Build history of the part. All positions in model axes, mm. A direction names the side the tool comes from. Coordinates: 2 decimals unless noted, no trailing zeros. Order: outer loops, then holes, each group sorted by start corner. A loop starts at its lowest first (then second) coordinate and runs counter-clockwise, first axis right, second up. Notation, with made-up numbers: (52.5, -30) - (102.5, -30) arc R33 ccw to (102.5, -1) - close; hole circle Ø1 at (82.25, -35.75). An arc over 180 degrees is marked (long way). Return JSON: item names as keys, results as strings.
from build123d import *

# Parameters (mm, degrees)
BOSS_EXTRUDE1_DEPTH      = 203.2
BOSS_EXTRUDE1_DEPTH_BACK = 203.2
SKETCH1_W                = 25.4
SKETCH1_H                = 25.4
SKETCH1_W_2              = 22.225
SKETCH1_H_2              = 22.225
FILLET1_R                = 0.79375
CUT_EXTRUDE1_DEPTH       = 206.174779152


with BuildPart() as part:
    # Sketch1 → Boss-Extrude1 (new, two sides: drawn at the far end of the back side and taken through both)
    with BuildSketch(Plane.XY.offset(-BOSS_EXTRUDE1_DEPTH_BACK)):
        Rectangle(SKETCH1_W, SKETCH1_H)
        Rectangle(SKETCH1_W_2, SKETCH1_H_2, mode=Mode.SUBTRACT)
    extrude(amount=BOSS_EXTRUDE1_DEPTH + BOSS_EXTRUDE1_DEPTH_BACK)

    # Fillet1
    fillet1_edges = [part.edges().sort_by_distance(p)[0] for p in [
        (12.7, -12.7, 0),
        (-12.7, -12.7, 0),
        (-12.7, 12.7, 0),
        (12.7, 12.7, 0),
    ]]
    fillet(fillet1_edges, radius=FILLET1_R)

    # Sketch3 → Cut-Extrude1 (cut, through all)
    with BuildSketch(Plane(origin=(12.7, 0, 0), x_dir=(0, 0, -1), z_dir=(1, 0, 0))):
        with BuildLine():
            Line((0, 3.2639), (203.2, 3.2639))
            ThreePointArc((203.2, 3.2639), (206.4639, 0), (203.2, -3.2639))
            Line((203.2, -3.2639), (0, -3.2639))
            ThreePointArc((0, -3.2639), (-3.2639, 0), (0, 3.2639))
        make_face()
    extrude(amount=-CUT_EXTRUDE1_DEPTH, mode=Mode.SUBTRACT)


solid = part.part
1. Probe L1, parallel to Y at x = 6, z = 140.5; L2, parallel to Y at x = 11.5, z = -149. List the from-to ranges inside material, lowest first.
Check values:
{"L1": "-12.7 to -11.11, 11.11 to 12.7", "L2": "-12.7 to -3.26, 3.26 to 12.7"}
2. Cut at A-A on y = 0. Give the cut face in (x, z), plus the area to 3 significant figures.
Check values:
{"outline": "(-12.7, 3.26) - (-11.11, 3.26) - (-11.11, 203.2) - (-12.7, 203.2) - close; (11.11, 3.26) - (12.7, 3.26) - (12.7, 203.2) - (11.11, 203.2) - close", "area": "635 mm²"}
3. Cut at D-D on z = 168. Give the cut face in (x, y), plus the area to 3 significant figures.
Check values:
{"outline": "(-12.7, -11.91) arc R0.79 ccw to (-11.91, -12.7) - (11.91, -12.7) arc R0.79 ccw to (12.7, -11.91) - (12.7, 11.91) arc R0.79 ccw to (11.91, 12.7) - (-11.91, 12.7) arc R0.79 ccw to (-12.7, 11.91) - close; hole (-11.11, -11.11) - (11.11, -11.11) - (11.11, 11.11) - (-11.11, 11.11) - close", "area": "151 mm²"}
4. Drop a flat-ended pin along its axis: pin 1 (1.7 mm diameter, centred on x = 12, z = -106.5, fed in from -Y). Give the stop position or say it passes through.
Check values:
{"pin 1": "y = -12.7"}
5. Mould opens along Y. For faces 3 (the flat face through (12.7, -5, -3)), 4 (the flat face through (0, 12.7, -3)), 5 (the flat face through (11.112, 5, -3)) say: pulls with the +Y half, pulls with the -Y half, needs draft (parallel to the pull), parting line crosses it, or undercut.
Check values:
{"face 3": "needs draft", "face 4": "pulls with the +Y half", "face 5": "undercut"}
6. Cut at B-B on x = 5.75. Give the cut face in (y, z), plus the area to 3 significant figures.
Check values:
{"outline": "(-12.7, -203.2) - (-11.11, -203.2) - (-11.11, 203.2) - (-12.7, 203.2) - close; (11.11, -203.2) - (12.7, -203.2) - (12.7, 203.2) - (11.11, 203.2) - close", "area": "1,290 mm²"}
7. Cut at C-C on z = -37. Give the cut face in (x, y), plus the area to 3 significant figures.
Check values:
{"outline": "(-12.7, -11.91) arc R0.79 ccw to (-11.91, -12.7) - (11.91, -12.7) arc R0.79 ccw to (12.7, -11.91) - (12.7, -3.26) - (11.11, -3.26) - (11.11, -11.11) - (-11.11, -11.11) - (-11.11, -3.26) - (-12.7, -3.26) - close; (-12.7, 3.26) - (-11.11, 3.26) - (-11.11, 11.11) - (11.11, 11.11) - (11.11, 3.26) - (12.7, 3.26) - (12.7, 11.91) arc R0.79 ccw to (11.91, 12.7) - (-11.91, 12.7) arc R0.79 ccw to (-12.7, 11.91) - close", "area": "130 mm²"}
8. Tool access for faces 1 (the flat face through (0, 11.112, -3)), 2 (the flat face through (-12.7, -5, -3)): list every direction of +Z, -Z, +X, -X, +Y, -Y with a clear straight run to the whole face (end or side of a thin tool).
Check values:
{"face 1": "+Z, -Z", "face 2": "+Z, -Z, -X, +Y, -Y"}
